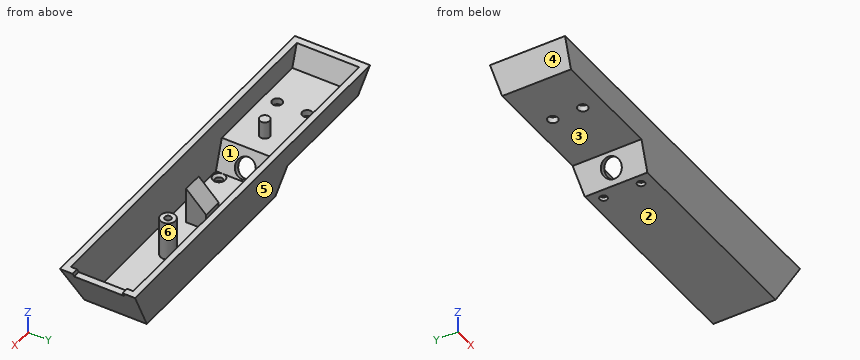
from build123d import *

# Parameters (mm, degrees)
PAD001_DEPTH      = 15
POCKET_DEPTH      = 75.001
POCKET_DEPTH_BACK = 75.001
THICKNESS_T       = -2.5
SKETCH006_R       = 3
PAD005_DEPTH      = 15.6
SKETCH007_R       = 1.3
POCKET001_DEPTH   = 15
SKETCH018_R       = 4
POCKET008_DEPTH   = 2.5
SKETCH020_R       = 2
POCKET009_DEPTH   = 12.501
SKETCH021_R       = 2
PAD008_DEPTH      = 7
SKETCH027_R       = 1.5
POCKET014_DEPTH   = 2.501
CHAMFER001_SIZE   = 1
SKETCH028_W       = 10
SKETCH028_H       = 20
POCKET015_DEPTH   = 2
SKETCH032_W       = 8
SKETCH032_H       = 8
PAD011_DEPTH      = 15
POCKET018_DEPTH   = 8


with BuildPart() as part:
    # Sketch001 → Pad001 (new body, symmetric)
    with BuildSketch(Plane.XZ):
        Polygon((-75, 0), (-69.2264973081, -10), (-24.2264973081, -10), (-18.4529946162, -20), (63.4529946162, -20), (75, 0), align=None)
    extrude(amount=PAD001_DEPTH, both=True)

    # Sketch002 → Pocket (cut, two sides)
    with BuildSketch(Plane.YZ) as pocket_sk:
        Polygon((-15, 0), (-12.5, -20), (-15, -20), align=None)
        Polygon((15, -20), (15, 0), (12.5, -20), align=None)
    extrude(amount=-POCKET_DEPTH, mode=Mode.SUBTRACT)
    extrude(pocket_sk.sketch, amount=POCKET_DEPTH_BACK, mode=Mode.SUBTRACT)

    # Thickness
    thickness_openings = [part.faces().sort_by_distance(p)[0] for p in [
        (0, 0, 0),
    ]]
    offset(amount=THICKNESS_T, openings=thickness_openings, kind=Kind.INTERSECTION)

    # Sketch006 (on Face14 of Thickness) → Pad005 (join)
    with BuildSketch(Plane.XY.offset(-17.5)):
        with Locations((30.0096189432, 0)):
            Circle(SKETCH006_R)
    extrude(amount=PAD005_DEPTH)

    # Sketch007 (on Face17 of Pad005) → Pocket001 (cut)
    with BuildSketch(Plane.XY.offset(-1.9)):
        with Locations((30.0096189432, 0)):
            Circle(SKETCH007_R)
    extrude(amount=-POCKET001_DEPTH, mode=Mode.SUBTRACT)

    # Sketch018 (on Face8 of Pocket001) → Pocket008 (cut)
    with BuildSketch(Plane(origin=(-22.5, 0, -12.9903810568), x_dir=(0, -1, 0), z_dir=(-0.8660254038, 0, -0.5))):
        with Locations((0, -2)):
            Circle(SKETCH018_R)
    extrude(amount=-POCKET008_DEPTH, mode=Mode.SUBTRACT)

    # Sketch020 (on Face14 of Pocket008) → Pocket009 (cut, through all)
    with BuildSketch(Plane.XY.offset(-7.5)):
        with Locations((-49.2831216351, 6)):
            Circle(SKETCH020_R)
        with Locations((-49.2831216351, -6)):
            Circle(SKETCH020_R)
    extrude(amount=-POCKET009_DEPTH, mode=Mode.SUBTRACT)

    # Sketch021 (on Face16 of Pocket009) → Pad008 (join)
    with BuildSketch(Plane.XY.offset(-7.5)):
        with Locations((-31.7831216351, 0)):
            Circle(SKETCH021_R)
    extrude(amount=PAD008_DEPTH)

    # Sketch027 (on Face18 of Pad008) → Pocket014 (cut, through all)
    with BuildSketch(Plane.XY.offset(-17.5)):
        with Locations((-14.5, 7.5)):
            Circle(SKETCH027_R)
        with Locations((-14.5, -7.5)):
            Circle(SKETCH027_R)
    extrude(amount=-POCKET014_DEPTH, mode=Mode.SUBTRACT)

    # Chamfer001
    chamfer001_edges = [part.edges().sort_by_distance(p)[0] for p in [
        (-16, 7.5, -17.5),
        (-16, -7.5, -17.5),
    ]]
    chamfer(chamfer001_edges, length=CHAMFER001_SIZE)

    # Sketch028 (on Face18 of Chamfer001) → Pocket015 (cut)
    with BuildSketch(Plane.XY):
        with Locations((70, 0)):
            Rectangle(SKETCH028_W, SKETCH028_H)
    extrude(amount=-POCKET015_DEPTH, mode=Mode.SUBTRACT)

    # Sketch032 (on Face4 of Pocket015) → Pad011 (join)
    with BuildSketch(Plane.XY.offset(-17.5)):
        with Locations((8, 0)):
            Rectangle(SKETCH032_W, SKETCH032_H)
    extrude(amount=PAD011_DEPTH)

    # Sketch033 (on Face17 of Pad011) → Pocket018 (cut)
    with BuildSketch(Plane.YZ.offset(12)):
        Polygon((4, -11), (-4, -3), (-4, -2.5), (4, -2.5), align=None)
    extrude(amount=-POCKET018_DEPTH, mode=Mode.SUBTRACT)


solid = part.part
Work out the finished part from the listing and answer in its coordinate system (mm). Face numbers are marked on the shaded views. A direction names the side the tool comes from. Give positions to 0.01 mm unless a question says otherwise; leave off trailing zeros. Loops run counter-clockwise (first coordinate to the right, second up) from the corner with the lowest first, then second, coordinate; pieces in that order, holes last. Notation, with made-up numbers: M 33.25,36 L 83.25,36 A20 ccw 83.25,66 Z; hole C 69,40 d4. An arc over 180 degrees is marked long. Use CSV: the item, a comma, the result in double quotes.
1) Find section A-A on x = -14.5. Write down the section's boundary in (y, z).
Answer:
outline,"M -15,0 L -12.5,-20 L -9,-20 L -9,-18.5 L -10,-17.5 L -10.29,-17.5 L -12.48,0 Z; M -6,-20 L 6,-20 L 6,-18.5 L 5,-17.5 L -5,-17.5 L -6,-18.5 Z; M 9,-20 L 12.5,-20 L 15,0 L 12.48,0 L 10.29,-17.5 L 10,-17.5 L 9,-18.5 Z"
2) Find section B-B on x = -58. Write down the section's boundary in (y, z), plus the area to 3 significant figures.
Answer:
outline,"M -15,0 L -13.75,-10 L 13.75,-10 L 15,0 L 12.48,0 L 11.54,-7.5 L -11.54,-7.5 L -12.48,0 Z"
area,"107 mm^2"
3) Determine the mould class of the marked faces 4, 5 and 6 for opening direction Y: released by +Y, released by -Y, zero draft, split by the parting line, or undercut.
Answer:
face 4,"zero draft"
face 5,"released by +Y"
face 6,"undercut"
4) Which of the six approach directions +Z, -Z, +X, -X, +Y, -Y give full straight-line access (tool end or side, diameter ignored) to the marked faces 1, 2 and 3?
Answer:
face 1,"+Z"
face 2,"-Z, +X, -X, +Y, -Y"
face 3,"-Z, -X, +Y, -Y"
5) Consider L1, parallel to Y at x = -14.5, z = -19.1; L2, parallel to X at y = -1.5, z = -2.5; L3, parallel to X at y = 2, z = -9.25. Determine where each line is inside the solid, lowest interval first.
Answer:
L1,"-12.61 to -9, -6 to 6, 9 to 12.61"
L2,"-73.56 to -70.67, -33.11 to -30.46, 27.41 to 32.61, 70.67 to 73.56"
L3,"-69.66 to -21.77, 4 to 12, 27.77 to 32.25, 66.77 to 69.66"
6) Given P1, Ø5, axis at x = -49.28, y = -6, coming from the +Z side; P2, Ø3, axis at x = 72, y = 2.5, coming from the +Z side; P3, Ø1, axis at y = 7.5, z = -16.5, coming from the -X side; P4, Ø2.5, axis at x = -14.5, y = 7.5, coming from the -Z side, each flat-ended and moving along its own axis, determine where each tip first touches the part or whether it passes through.
Answer:
P1,"z = -7.5"
P2,"z = -2"
P3,"x = -20.76"
P4,"through"
